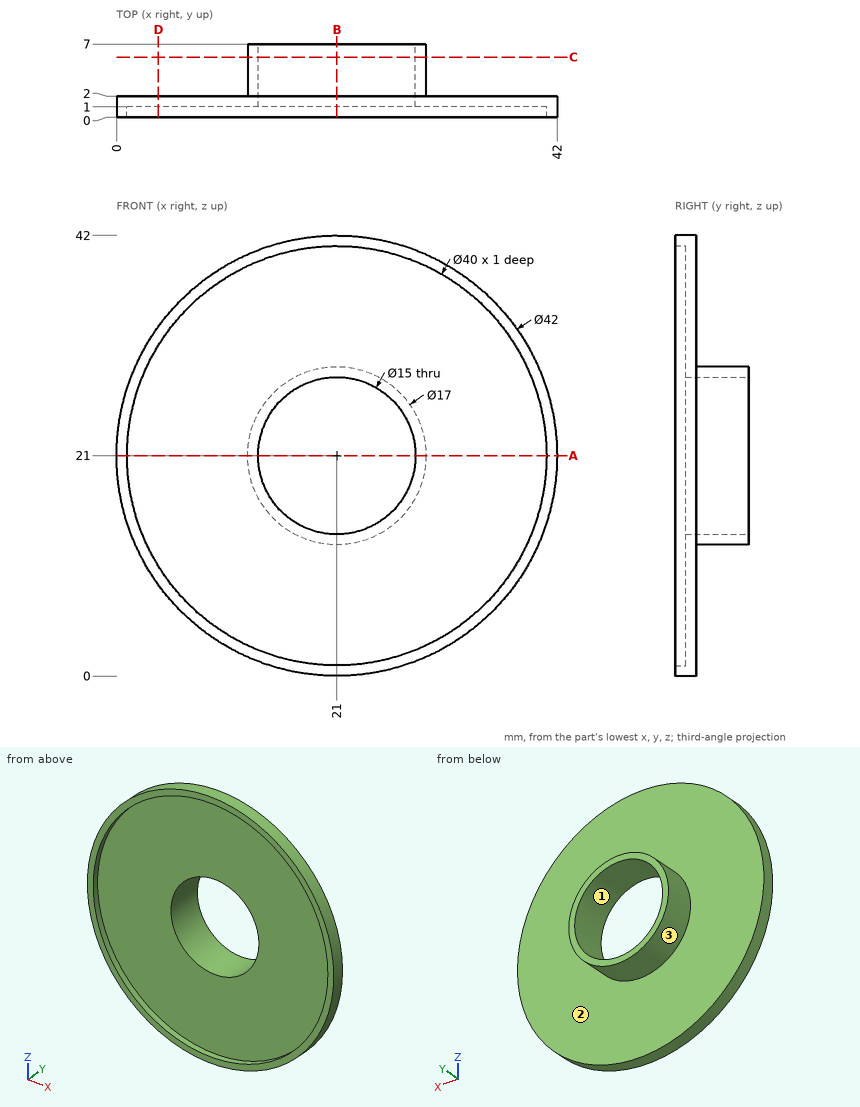
Here's the drawing with two shaded views (mm, measured from the low corner). I have some questions. Round coordinates to 2 decimals unless told otherwise and drop trailing zeros. Loops run counter-clockwise (first coordinate to the right, second up) from the corner with the lowest first, then second, coordinate; pieces in that order, holes last. Notation, with made-up numbers: (17, -31.75) - (26, -31.75) arc R22 cw to (26, -14.75) - close; hole circle Ø4 at (-36.75, 6.25). An arc over 180 degrees is marked (long way). Use CSV: the item, a comma, the result in double quotes. Start each with the question number.
1) If we section it at B-B on x = 21: Write out the boundary of the cut face in (y, z), plus the area to 3 significant figures.
2) We'd pull the mould along X, two halves only. Please class the marked faces 1, 2 and 3: released by +X, released by -X, zero draft, split by the parting line, or undercut.
3) Please list where these lines run through material, in increasing order: probe 1 along X at (y, z) = (5.7, 21); probe 2 along X at (y, z) = (0.4, 21). Write a range as [from, to].
4) If we section it at D-D on x = 4: Write out the boundary of the cut face in (y, z).
5) If we section it at A-A on z = 21: Write out the boundary of the cut face in (x, y), plus the area to 3 significant figures.
6) For pin 1 Ø4 at (y, z) = (1, 24.5) entering from -X; pin 2 Ø1 at (y, z) = (5.5, 14) entering from +X; pin 3 Ø3 at (x, y) = (35, 4) entering from +Z; pin 4 Ø1.5 at (x, y) = (26, 6) entering from +Z, each with a flat end and sliding along its axis, tell me the tip position at first contact or that it passes through.
7) If we section it at C-C on y = 5.75: Write out the boundary of the cut face in (x, z), plus the area to 3 significant figures.
Geometry results:
1,outline,"(0, 0) - (2, 0) - (2, 12.5) - (7, 12.5) - (7, 13.5) - (1, 13.5) - (1, 1) - (0, 1) - close; (0, 41) - (1, 41) - (1, 28.5) - (7, 28.5) - (7, 29.5) - (2, 29.5) - (2, 42) - (0, 42) - close"
1,area,"39.0 mm2"
2,face 1,"undercut"
2,face 2,"zero draft"
2,face 3,"split by the parting line"
3,probe 1,"x = [12.5, 13.5], [28.5, 29.5]"
3,probe 2,"x = [0, 1], [41, 42]"
4,outline,"(0, 8.67) - (2, 8.67) - (2, 33.33) - (0, 33.33) - (0, 31.54) - (1, 31.54) - (1, 10.46) - (0, 10.46) - close"
5,outline,"(0, 0) - (1, 0) - (1, 1) - (13.5, 1) - (13.5, 7) - (12.5, 7) - (12.5, 2) - (0, 2) - close; (28.5, 1) - (41, 1) - (41, 0) - (42, 0) - (42, 2) - (29.5, 2) - (29.5, 7) - (28.5, 7) - close"
5,area,"39.0 mm2"
6,pin 1,"stops at x = 0.05"
6,pin 2,"stops at x = 26.48"
6,pin 3,"passes through"
6,pin 4,"stops at z = 28.36"
7,outline,"circle Ø17 at (21, 21); hole circle Ø15 at (21, 21)"
7,area,"50.3 mm2"
